Geometry check sheet. Reference: the model listing, model coordinates, mm. Face numbers are marked on the shaded views. Give positions to 0.01 mm unless a question says otherwise; leave off trailing zeros. Write each loop counter-clockwise with the first axis right and the second up, starting at its lowest first coordinate (ties: lowest second). Pieces come first, ordered by that corner, then holes. Notation, with made-up numbers: M 29,61.25 L 39,61.25 A25 cw 39,93.25 Z; hole C 2,77 d5. An arc over 180 degrees is marked long. One line per item, written item: value. Start each with the question number.
1. Cross-section at B-B on x = 69.85. Record the cut outline in (y, z), then the cut area to 3 significant figures.
2. Scan lines: line 1 (Y direction, x = 5, z = 0.1); line 2 (Y direction, x = 44.45, z = 1); line 3 (Y direction, x = 74.5, z = 0.3). Record each from-to range of solid material in increasing order.
3. Cross-section at A-A on z = 0.8. Count the separate pieces of the cut face and the enclosed holes in it, then the cut area to 3 significant figures.
4. Release check for a two-part mould opening along Z. For the marked faces 1 and 2 record: pulls with the +Z half, pulls with the -Z half, needs draft (parallel to the pull), parting line crosses it, or undercut.
from build123d import *

# Parameters (mm, degrees)
SKETCH1_R           = 0.5
BOSS_EXTRUDE1_DEPTH = 1.6


with BuildPart() as part:
    # Sketch1 → Boss-Extrude1 (new body)
    with BuildSketch(Plane.XY.offset(1.6)):
        with BuildLine():
            Line((0, 53.320743496), (0, 3.473243496))
            ThreePointArc((0, 3.473243496), (0.697451977, 1.789445473), (2.38125, 1.091993496))
            Line((2.38125, 1.091993496), (58.7375, 1.091993496))
            ThreePointArc((58.7375, 1.091993496), (59.860032015, 1.556961481), (60.325, 2.679493496))
            ThreePointArc((60.325, 2.679493496), (69.85, 12.204493496), (79.375, 2.679493496))
            ThreePointArc((79.375, 2.679493496), (79.839967985, 1.556961481), (80.9625, 1.091993496))
            Line((80.9625, 1.091993496), (86.51875, 1.091993496))
            ThreePointArc((86.51875, 1.091993496), (88.202548023, 1.789445473), (88.9, 3.473243496))
            Line((88.9, 3.473243496), (88.9, 53.320743496))
            ThreePointArc((88.9, 53.320743496), (88.202548023, 55.004541519), (86.51875, 55.701993496))
            Line((86.51875, 55.701993496), (2.38125, 55.701993496))
            ThreePointArc((2.38125, 55.701993496), (0.697451977, 55.004541519), (0, 53.320743496))
        make_face()
        with Locations((4.7625, 50.939493496)):
            Circle(SKETCH1_R, mode=Mode.SUBTRACT)
        with Locations((4.7625, 5.854493496)):
            Circle(SKETCH1_R, mode=Mode.SUBTRACT)
        with Locations((84.1375, 5.854493496)):
            Circle(SKETCH1_R, mode=Mode.SUBTRACT)
        with Locations((84.1375, 50.939493496)):
            Circle(SKETCH1_R, mode=Mode.SUBTRACT)
        with Locations((30.559375, 5.854493496)):
            Circle(SKETCH1_R, mode=Mode.SUBTRACT)
        with Locations((55.5625, 5.854493496)):
            Circle(SKETCH1_R, mode=Mode.SUBTRACT)
        with Locations((44.45, 50.939493496)):
            Circle(SKETCH1_R, mode=Mode.SUBTRACT)
    extrude(amount=-BOSS_EXTRUDE1_DEPTH)


solid = part.part
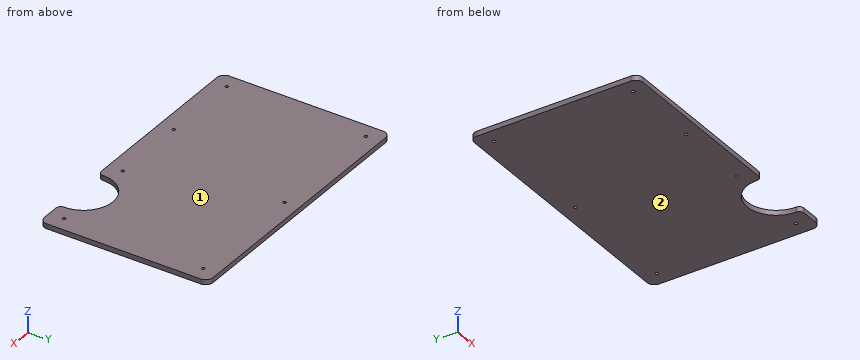
Report:
1. outline: M 12.2,0 L 55.7,0 L 55.7,1.6 L 12.2,1.6 Z
1. area: 69.6 mm^2
2. line 1: y = 1.09 to 5.41, 6.29 to 50.5, 51.38 to 55.7
2. line 2: y = 1.09 to 50.44, 51.44 to 55.7
2. line 3: y = 10.99 to 55.7
3. separate pieces: 1
3. enclosed holes: 7
3. area: 4,670 mm^2
4. face 1: pulls with the +Z half
4. face 2: pulls with the -Z half
